For this review, take the finished solid that the model builds, in its own axes (mm). A direction names the side the tool comes from. Give positions to 0.01 mm unless a question says otherwise; leave off trailing zeros. Write each loop counter-clockwise with the first axis right and the second up, starting at its lowest first coordinate (ties: lowest second). Pieces come first, ordered by that corner, then holes.
from build123d import *

# Parameters (mm, degrees)
F0_R     = 4.4958
F1_DEPTH = 24.13
F3_W     = 6.35
F3_H     = 21.166668
F4_DEPTH = 5.715
F5_SIZE  = 0.508
F7_W     = 18.438894
F7_H     = 4.169167
F8_DEPTH = 21.336
F10_D    = 4.0894


with BuildPart() as f1:
    # F0 (on Front) → F1 (new body)
    with BuildSketch(Plane.XZ):
        Circle(F0_R)
    extrude(amount=-F1_DEPTH)

    # F3 (on offset) → F4 (cut)
    with BuildSketch(Plane.XZ.offset(2.54)):
        with Locations((-5.588, -0.807043)):
            Rectangle(F3_W, F3_H)
        with Locations((5.588, -0.807043)):
            Rectangle(F3_W, F3_H)
    extrude(amount=-F4_DEPTH, mode=Mode.SUBTRACT)

    # F5
    f5_edges = [f1.edges().sort_by_distance(p)[0] for p in [
        (-2.413, 0, 0),
        (2.413, 0, 0),
    ]]
    chamfer(f5_edges, length=F5_SIZE)

    # F7 (on offset) → F8 (cut)
    with BuildSketch(Plane(origin=(0, 26.67, 0), x_dir=(1, 0, 0), z_dir=(0, 1, 0))):
        with Locations((-0.012653, 5.259583)):
            Rectangle(F7_W, F7_H)
        with Locations((-0.012653, -5.259583)):
            Rectangle(F7_W, F7_H)
    extrude(amount=-F8_DEPTH, mode=Mode.SUBTRACT)

    # F10 (through all)
    with Locations(Plane.XZ):
        with Locations((0, 0)):
            Hole(F10_D / 2)


solid = f1.part
(1) We need section B-B (z = 1.75). Write out the cut boundary in (x, y) (1 decimal), and give its area (3 significant figures).
(2) Tool access review of faces 4 (the flat face through (0, 15, 3.175)), 5 (the flat face through (0, 15, -3.175)), 6 (the flat face through (2.413, 2, 0)): name each direction out of +Z, -Z, +X, -X, +Y, -Y from which nothing blocks a thin tool from reaching the whole face with its end or side.
(3) For L1, parallel to Z at x = 0, y = 17.5 (3 decimals); L2, parallel to X at y = 9.5, z = 0; L3, parallel to X at y = 20.5, z = -1, list the stretches that pass through material, from the lowest coordinate up.
(4) We need section C-C (y = 8.75). Write out the cut boundary in (x, z) (3 decimals).
(5) We need section A-A (x = 0). Write out the cut boundary in (y, z) (3 decimals).
(6) We need section D-D (z = 2.75). Write out the cut boundary in (x, y) (3 decimals), and give its area (3 significant figures).
(7) Clearance check with flat-ended pins moving along their axes: pin 1 Ø1.5 at (x, y) = (3.5, 19) entering from +Z (3 decimals); pin 2 Ø1.3 at (y, z) = (1.5, 1.5) entering from +X; pin 3 Ø1.7 at (x, z) = (3.5, -0.5) entering from -Y (3 decimals). State where each tip first meets the part, or that it passes through.
(8) The part is to be moulded in two halves that separate along X. For faces 1 (the flat face through (0, 0, -3)), 2 (the flat face through (-2.413, 2, 0)), 3 (the cylindrical face through (-1.95, 12.23, 0.61)), say which applies: +X half, -X half, draft (parallel to the pull), parting line (faces both ways), or undercut.
The answers:
1. outline: (-4.1, 3.2) - (-2.4, 3.2) - (-2.4, 0.5) - (-1.9, 0) - (-1.1, 0) - (-1.1, 24.1) - (-4.1, 24.1) - close; (1.1, 0) - (1.9, 0) - (2.4, 0.5) - (2.4, 3.2) - (4.1, 3.2) - (4.1, 24.1) - (1.1, 24.1) - close
1. area: 138 mm2
2. face 4: +Z, +X, -X, +Y
2. face 5: -Z, +X, -X, +Y
2. face 6: +Z, -Z, +X, -Y
3. L1: z = -3.175 to -2.045, 2.045 to 3.175
3. L2: x = -4.5 to -2.04, 2.04 to 4.5
3. L3: x = -4.38 to -1.78, 1.78 to 4.38
4. outline: (-3.183, -3.175) - (3.183, -3.175) arc R4.496 ccw to (3.183, 3.175) - (-3.183, 3.175) arc R4.496 ccw to start; hole circle Ø4.089 at (0, 0)
5. outline: (0, -4.496) - (5.334, -4.496) - (5.334, -3.175) - (24.13, -3.175) - (24.13, -2.045) - (0, -2.045) - close; (0, 2.045) - (24.13, 2.045) - (24.13, 3.175) - (5.334, 3.175) - (5.334, 4.496) - (0, 4.496) - close
6. outline: (-3.557, 3.175) - (-2.413, 3.175) - (-2.413, 0.508) - (-1.905, 0) - (1.905, 0) - (2.413, 0.508) - (2.413, 3.175) - (3.557, 3.175) - (3.557, 24.13) - (-3.557, 24.13) - close
6. area: 164 mm2
7. pin 1: stops at z = 3.175
7. pin 2: stops at x = 2.41
7. pin 3: stops at y = 3.175
8. face 1: draft
8. face 2: -X half
8. face 3: undercut
